```python
from build123d import *

# Parameters (mm, degrees)
SKETCH1_W           = 20.240625
SKETCH1_H           = 21.828125
BOSS_EXTRUDE1_DEPTH = 20.32
CUT_EXTRUDE1_DEPTH  = 20.32
SKETCH4_W           = 20.240625
SKETCH4_H           = 20.32
BOSS_EXTRUDE2_DEPTH = 4.445
BOSS_EXTRUDE3_DEPTH = 2.54
BOSS_EXTRUDE4_DEPTH = 2.54
SKETCH8_W           = 16.35125
SKETCH8_H           = 25.4
BOSS_EXTRUDE5_DEPTH = 7.62
SKETCH10_R          = 1.27
CUT_EXTRUDE3_DEPTH  = 35.580044657
CUT_EXTRUDE4_DEPTH  = 25.4
SKETCH14_W          = 16.35125
SKETCH14_H          = 25.4
CUT_EXTRUDE5_DEPTH  = 3.81


with BuildPart() as part:
    # Sketch1 → Boss-Extrude1 (new body)
    with BuildSketch(Plane(origin=(0, 0, 0), x_dir=(1, 0, 0), z_dir=(0, 1, 0))):
        Rectangle(SKETCH1_W, SKETCH1_H)
    extrude(amount=BOSS_EXTRUDE1_DEPTH)

    # Sketch2 → Cut-Extrude1 (cut)
    with BuildSketch(Plane(origin=(0, 20.32, 0), x_dir=(1, 0, 0), z_dir=(0, 1, 0))):
        Polygon((10.1203125, 0.9921875), (3.7703125, 0.9921875), (3.7703125, 5.7546875), (9.1203125, 5.7546875), (9.1203125, 8.5328125), (6.9453125, 8.5328125), (6.9453125, 10.9140625), (10.1203125, 10.9140625), (10.1203125, 8.5328125), (10.1203125, 5.7546875), align=None)
        Polygon((-6.9453125, 10.9140625), (-10.1203125, 10.9140625), (-10.1203125, 8.5328125), (-10.1203125, 5.7546875), (-10.1203125, 0.9921875), (-3.7703125, 0.9921875), (-3.7703125, 5.7546875), (-9.1203125, 5.7546875), (-9.1203125, 8.5328125), (-6.9453125, 8.5328125), align=None)
    extrude(amount=-CUT_EXTRUDE1_DEPTH, mode=Mode.SUBTRACT)

    # Sketch4 → Boss-Extrude2 (add)
    with BuildSketch(Plane.XY.offset(10.9140625)):
        with Locations((0, 10.16)):
            Rectangle(SKETCH4_W, SKETCH4_H)
    extrude(amount=BOSS_EXTRUDE2_DEPTH)

    # Sketch6 → Boss-Extrude3 (add)
    with BuildSketch(Plane(origin=(0, 20.32, 0), x_dir=(1, 0, 0), z_dir=(0, 1, 0))):
        Polygon((-10.1203125, -15.3590625), (-10.1203125, 0.9921875), (-3.7703125, 0.9921875), (-3.7703125, 5.7546875), (-9.1203125, 5.7546875), (-9.1203125, 8.5328125), (-6.9453125, 8.5328125), (-6.9453125, 10.9140625), (6.9453125, 10.9140625), (6.9453125, 8.5328125), (9.1203125, 8.5328125), (9.1203125, 5.7546875), (3.7703125, 5.7546875), (3.7703125, 0.9921875), (10.1203125, 0.9921875), (10.1203125, -15.3590625), align=None)
    extrude(amount=BOSS_EXTRUDE3_DEPTH)

    # Sketch7 → Boss-Extrude4 (add)
    with BuildSketch(Plane.XZ):
        Polygon((-10.1203125, -0.9921875), (-10.1203125, 15.3590625), (10.1203125, 15.3590625), (10.1203125, -0.9921875), (3.7703125, -0.9921875), (3.7703125, -5.7546875), (9.1203125, -5.7546875), (9.1203125, -8.5328125), (6.9453125, -8.5328125), (6.9453125, -10.9140625), (-6.9453125, -10.9140625), (-6.9453125, -8.5328125), (-9.1203125, -8.5328125), (-9.1203125, -5.7546875), (-3.7703125, -5.7546875), (-3.7703125, -0.9921875), align=None)
    extrude(amount=BOSS_EXTRUDE4_DEPTH)

    # Sketch8 → Boss-Extrude5 (add)
    with BuildSketch(Plane(origin=(10.1203125, 0, 0), x_dir=(0, 0, -1), z_dir=(1, 0, 0))):
        with Locations((-7.1834375, 10.16)):
            Rectangle(SKETCH8_W, SKETCH8_H)
    extrude(amount=BOSS_EXTRUDE5_DEPTH)

    # Sketch10 → Cut-Extrude3 (cut, through all)
    with BuildSketch(Plane.XZ.offset(2.54)):
        with Locations(Location((5.1196875, 3.0718125, 0), (0, 0, 270))):
            Circle(SKETCH10_R)
    extrude(amount=-CUT_EXTRUDE3_DEPTH, mode=Mode.SUBTRACT)

    # Sketch12 → Cut-Extrude4 (cut)
    with BuildSketch(Plane(origin=(17.7403125, 0, 0), x_dir=(0, 0, -1), z_dir=(1, 0, 0))):
        Polygon((-15.3590625, 18.034), (-15.3590625, 2.286), (-11.5490625, 2.286), (-11.5490625, 3.556), (-6.7230625, 3.556), (-6.7230625, 2.286), (-1.3890625, 2.286), (-1.3890625, 18.034), (-6.7230625, 18.034), (-6.7230625, 16.764), (-11.5490625, 16.764), (-11.5490625, 18.034), align=None)
    extrude(amount=-CUT_EXTRUDE4_DEPTH, mode=Mode.SUBTRACT)

    # Sketch14 → Cut-Extrude5 (cut)
    with BuildSketch(Plane(origin=(17.7403125, 0, 0), x_dir=(0, 0, -1), z_dir=(1, 0, 0))):
        with Locations((-7.1834375, 10.16)):
            Rectangle(SKETCH14_W, SKETCH14_H)
    extrude(amount=-CUT_EXTRUDE5_DEPTH, mode=Mode.SUBTRACT)


solid = part.part
```
CAD build for the part. Positions are in the model's coordinates, mm. A direction names the side the tool comes from. Give positions to 0.01 mm unless a question says otherwise; leave off trailing zeros. Order: outer loops, then holes, each group sorted by start corner. A loop starts at its lowest first (then second) coordinate and runs counter-clockwise, first axis right, second up.
(1) Tool access for faces 4 (the flat face through (6, 10, -5.755)), 5 (the flat face through (9.12, 10, -7)), 6 (the flat face through (-6.945, 10, -10)): list every direction of +Z, -Z, +X, -X, +Y, -Y with a clear straight run to the whole face (end or side of a thin tool).
(2) Saw through at C-C, the plane y = 16. Give the cut face in (x, z).
(3) Flat gauge pins, fed straight in: pin 1 (4.5 mm diameter, centred on x = 7.5, y = 14, fed in from +Z); pin 2 (1.4 mm diameter, centred on y = 7, z = -3, fed in from +X); pin 3 (1.4 mm diameter, centred on y = 4.5, z = -7, fed in from +X). Where does each tip first touch, or does it go through?
(4) Saw through at A-A, the plane x = -5. Give the cut face in (y, z).
(5) Saw through at B-B, the plane z = 2.75. Give the cut face in (x, y), then the cut area to 3 significant figures.
(6) Drill centre lines: L1, parallel to Z at x = -6.25, y = 2; L2, parallel to Y at x = 7.5, z = 6; L3, parallel to Z at x = 8.75, y = 5.75. Where is each one in solid material? Low to high.
(7) Saw through at D-D, the plane x = 10.75. Give the cut face in (y, z).
(8) Mould opens along X. For faces 1 (the flat face through (9, 10, -0.992)), 2 (the flat face through (-3.77, 10, -3)), 3 (the cylindrical face through (6.19, -0.16, 2.39)) say: released by +X, released by -X, zero draft, split by the parting line, or undercut.
Results found:
1. face 4: +X, +Y, -Y
1. face 5: -Z, +X, +Y, -Y
1. face 6: -Z, -X, +Y, -Y
2. outline: (-10.12, -0.99) - (-3.77, -0.99) - (-3.77, -5.75) - (-9.12, -5.75) - (-9.12, -8.53) - (-6.95, -8.53) - (-6.95, -10.91) - (6.95, -10.91) - (6.95, -8.53) - (9.12, -8.53) - (9.12, -5.75) - (3.77, -5.75) - (3.77, -0.99) - (13.93, -0.99) - (13.93, 1.39) - (-7.66, 1.39) - (-7.66, 15.36) - (-10.12, 15.36) - close
3. pin 1: stops at z = 1.39
3. pin 2: stops at x = 3.77
3. pin 3: stops at x = 9.12
4. outline: (-2.54, -10.91) - (22.86, -10.91) - (22.86, -5.75) - (-2.54, -5.75) - close; (-2.54, -0.99) - (22.86, -0.99) - (22.86, 15.36) - (18.03, 15.36) - (18.03, 11.55) - (16.76, 11.55) - (16.76, 6.72) - (18.03, 6.72) - (18.03, 1.39) - (2.29, 1.39) - (2.29, 6.72) - (3.56, 6.72) - (3.56, 11.55) - (2.29, 11.55) - (2.29, 15.36) - (-2.54, 15.36) - close
5. outline: (-10.12, -2.54) - (3.89, -2.54) - (3.89, 2.29) - (-7.66, 2.29) - (-7.66, 18.03) - (3.89, 18.03) - (3.89, 22.86) - (-10.12, 22.86) - close; (6.35, -2.54) - (13.93, -2.54) - (13.93, 2.29) - (6.35, 2.29) - close; (6.35, 18.03) - (13.93, 18.03) - (13.93, 22.86) - (6.35, 22.86) - close
5. area: 247 mm2
6. L1: z = -10.91 to -5.75, -0.99 to 15.36
6. L2: y = -2.54 to 2.29, 18.03 to 22.86
6. L3: z = -8.53 to -5.75, -0.99 to 1.39
7. outline: (-2.54, -0.99) - (22.86, -0.99) - (22.86, 15.36) - (18.03, 15.36) - (18.03, 11.55) - (16.76, 11.55) - (16.76, 6.72) - (18.03, 6.72) - (18.03, 1.39) - (2.29, 1.39) - (2.29, 6.72) - (3.56, 6.72) - (3.56, 11.55) - (2.29, 11.55) - (2.29, 15.36) - (-2.54, 15.36) - close
8. face 1: zero draft
8. face 2: released by -X
8. face 3: undercut
